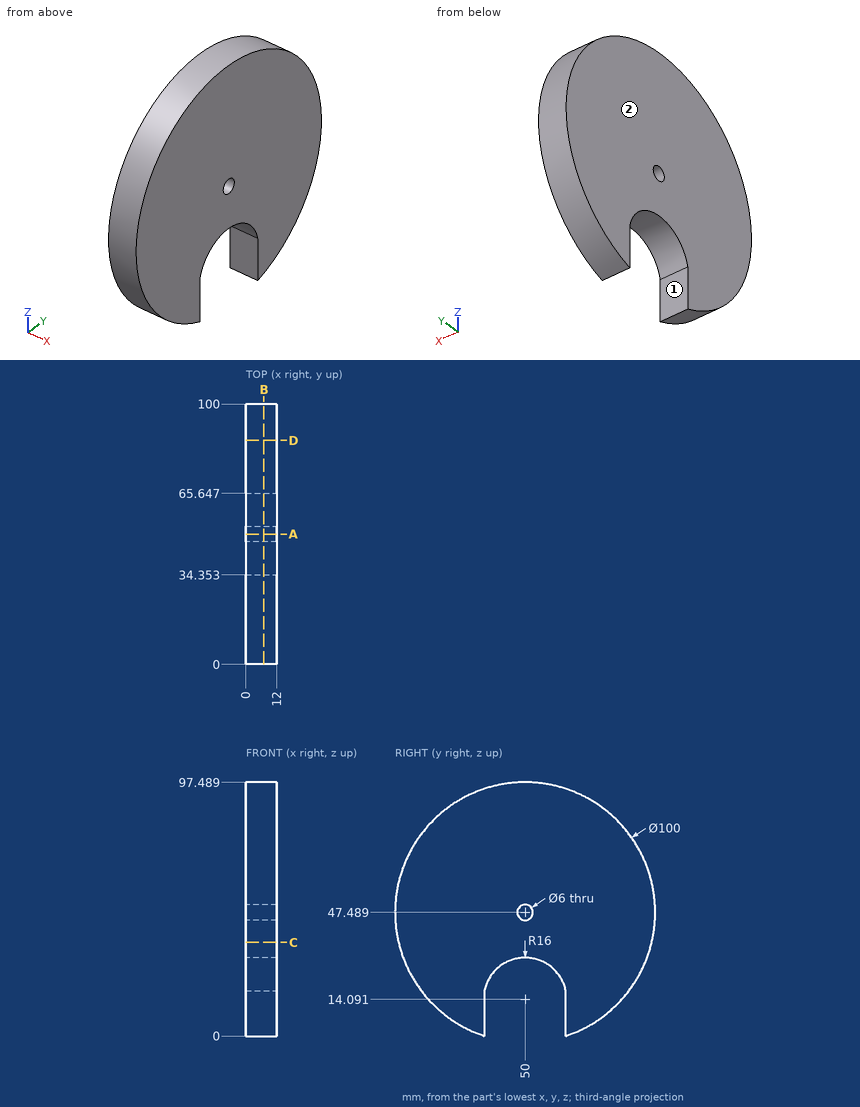
Part print with two shaded views. Sizes in mm from the minimum x, y, z corner. A direction names the side the tool comes from. Round coordinates to 2 decimals unless told otherwise and drop trailing zeros. Order: outer loops, then holes, each group sorted by start corner. A loop starts at its lowest first (then second) coordinate and runs counter-clockwise, first axis right, second up. Notation, with made-up numbers: (-4, 75.25) - (34, 75.25) arc R27 ccw to (34, 113.25) - close; hole circle Ø6 at (68.5, -26.5). An arc over 180 degrees is marked (long way). Answer in a Markdown table with one row per item. Add a question column.
(1) Band-saw the part on D-D on y = 86. List the corners of the cut face in (x, z), and give its area (3 significant figures).
(2) Band-saw the part on B-B on x = 7. List the corners of the cut face in (y, z) (1 decimal), and give its area (3 significant figures).
(3) Drop flat-ended pins along their axis: pin 1 Ø3.5 at (x, z) = (4, 7) entering from +Y; pin 2 Ø3 at (x, y) = (2.5, 43) entering from -Z (1 decimal); pin 3 Ø5 at (x, z) = (6.5, 17.5) entering from +Y (1 decimal). Give the stop position or say it passes through.
(4) Probe L1, parallel to Z at x = 9.25, y = 50; L2, parallel to Y at x = 7.5, z = 48 (1 decimal); L3, parallel to Y at x = 1.5, z = 27.5 (1 decimal). List the from-to ranges inside material, lowest first. Write a range as [from, to].
(5) Band-saw the part on A-A on y = 50. List the corners of the cut face in (x, z), and give its area (3 significant figures).
(6) 3-axis set-ups, long thin cutter, end or side, ignore diameter. For the marked faces 1 and 2: which of +Z, -Z, +X, -X, +Y, -Y reach the whole face in a straight line?
(7) Band-saw the part on C-C on z = 36. List the corners of the cut face in (x, y), and give its area (3 significant figures).
Data:
| question | item | result |
|---|---|---|
| 1 | outline | (0, 12.79) - (12, 12.79) - (12, 82.19) - (0, 82.19) - close |
| 1 | area | 833 mm^2 |
| 2 | outline | (34.4, 0) - (34.4, 17.4) arc R16 cw to (65.6, 17.4) - (65.6, 0) arc R50 ccw (long way) to start; hole circle Ø6 at (50, 47.5) |
| 2 | area | 6,930 mm^2 |
| 3 | pin 1 | stops at y = 81.61 |
| 3 | pin 2 | stops at z = 27.6 |
| 3 | pin 3 | stops at y = 91.8 |
| 4 | L1 | z = [30.09, 44.49], [50.49, 97.49] |
| 4 | L2 | y = [0, 47], [53, 100] |
| 4 | L3 | y = [4.2, 41.3], [58.7, 95.8] |
| 5 | outline | (0, 30.09) - (12, 30.09) - (12, 44.49) - (0, 44.49) - close; (0, 50.49) - (12, 50.49) - (12, 97.49) - (0, 97.49) - close |
| 5 | area | 737 mm^2 |
| 6 | face 1 | -Z, +X, -X |
| 6 | face 2 | +Z, -Z, -X, +Y, -Y |
| 7 | outline | (0, 1.34) - (12, 1.34) - (12, 98.66) - (0, 98.66) - close |
| 7 | area | 1,170 mm^2 |
